Build history of the part. All positions in model axes, mm. A direction names the side the tool comes from. Give positions to 0.01 mm unless a question says otherwise; leave off trailing zeros. Order: outer loops, then holes, each group sorted by start corner. A loop starts at its lowest first (then second) coordinate and runs counter-clockwise, first axis right, second up. Notation, with made-up numbers: (30.5, 46) - (61.5, 46) arc R21 cw to (61.5, 77) - close; hole circle Ø6 at (-24.5, 29.5). An arc over 180 degrees is marked (long way). One line per item, written item: value.
```python
from build123d import *

# Parameters (mm, degrees)
CYLINDER063_R              = 1.6
CYLINDER063_DEPTH          = 10
EXTRUDE027_DEPTH           = 6
EXTRUDE030_DEPTH           = 6
EXTRUDE030_PLACEMENT_ANGLE = 180
CYLINDER072_R              = 1.5
CYLINDER072_DEPTH          = 45
PRISM011_DEPTH             = 3
CYLINDER071_R              = 3
CYLINDER071_DEPTH          = 5
FUSION063_PLACEMENT_ANGLE  = 180
CYLINDER070_R              = 1.5
CYLINDER070_DEPTH          = 45
PRISM010_DEPTH             = 3
CYLINDER068_R              = 3
CYLINDER068_DEPTH          = 5
EXTRUDE026_DEPTH           = 24
REVOLVE001_ANGLE           = 180
EXTRUDE025_DEPTH           = 74
FILLET004_R                = 2.5


with BuildPart() as cono003:
    # Cone003 → Cone003 (revolve)
    with BuildSketch(Plane(origin=(0, 0, -96), x_dir=(1, 0, 0), z_dir=(0, -1, 0))):
        Polygon((0, 0), (1.6, 0), (4.1, 3), (0, 3), align=None)
    revolve(axis=Axis((0, 0, -96), (0, 0, 1)))


with BuildPart() as cilindro063:
    # Cylinder063 → Cylinder063 (new body)
    with BuildSketch(Plane.XY.offset(-106)):
        Circle(CYLINDER063_R)
    extrude(amount=CYLINDER063_DEPTH)


with BuildPart() as fusion058:
    # Fusion058 base: copy of Cilindro063
    add(cilindro063.part)

    # Fusion058: union Cono003
    add(cono003.part)


with BuildPart() as fusion058_1:
    # Fusion058 placement: moved
    add(fusion058.part.moved(Location((65, 107, 0))))


with BuildPart() as fusion059:
    # Fusion057 base: copy of Cilindro063
    add(cilindro063.part)

    # Fusion057: union Cono003
    add(cono003.part)


with BuildPart() as fusion059_1:
    # Fusion057 placement: moved
    add(fusion059.part.moved(Location((-65, 107, 0))))

    # Fusion059: union Fusion058
    add(fusion058_1.part)


with BuildPart() as extrude027:
    # Sketch020 → Extrude027 (new body)
    with BuildSketch(Plane.XY.offset(-99)):
        with BuildLine():
            ThreePointArc((0, 10), (-10, 0), (0, -10))
            Line((20, -10), (0, -10))
            Line((20, 10), (20, -10))
            Line((0, 10), (20, 10))
        make_face()
    extrude(amount=EXTRUDE027_DEPTH)


with BuildPart() as extrude027_1:
    # Extrude027 placement: moved
    add(extrude027.part.moved(Location((-65, 107, 0))))


with BuildPart() as cut022:
    # Sketch020 → Extrude030 (new body)
    with BuildSketch(Plane.XY.offset(-99)):
        with BuildLine():
            ThreePointArc((0, 10), (-10, 0), (0, -10))
            Line((20, -10), (0, -10))
            Line((20, 10), (20, -10))
            Line((0, 10), (20, 10))
        make_face()
    extrude(amount=EXTRUDE030_DEPTH)


with BuildPart() as cut022_1:
    # Extrude030 placement: moved
    add(cut022.part.moved(Location((65, 107, 0))).rotate(Axis((65, 107, 0), (0, 0, 1)), EXTRUDE030_PLACEMENT_ANGLE))

    # Fusion055: union Extrude027
    add(extrude027_1.part)

    # Cut022: cut Fusion059
    add(fusion059_1.part, mode=Mode.SUBTRACT)


with BuildPart() as cilindro072:
    # Cylinder072 → Cylinder072 (new body)
    with BuildSketch(Plane(origin=(33, 0, -87), x_dir=(0, 0, 1), z_dir=(-1, 0, 0))):
        Circle(CYLINDER072_R)
    extrude(amount=CYLINDER072_DEPTH)


with BuildPart() as prisma011:
    # Prism011 → Prism011 (new body)
    with BuildSketch(Plane(origin=(0, 0, -87), x_dir=(0, 0, 1), z_dir=(-1, 0, 0))):
        Polygon((3, 0), (1.5, 2.598076), (-1.5, 2.598076), (-3, 0), (-1.5, -2.598076), (1.5, -2.598076), align=None)
    extrude(amount=PRISM011_DEPTH)


with BuildPart() as fusion063:
    # Cylinder071 → Cylinder071 (new body)
    with BuildSketch(Plane(origin=(24, 0, -87), x_dir=(0, 0, 1), z_dir=(-1, 0, 0))):
        Circle(CYLINDER071_R)
    extrude(amount=CYLINDER071_DEPTH)

    # Fusion063: union Cilindro072, Prisma011
    add(cilindro072.part)
    add(prisma011.part)


with BuildPart() as fusion063_1:
    # Fusion063 placement: moved
    add(fusion063.part.moved(Location((-65, 36, 0))).rotate(Axis((-65, 36, 0), (0, 0, 1)), FUSION063_PLACEMENT_ANGLE))


with BuildPart() as cilindro070:
    # Cylinder070 → Cylinder070 (new body)
    with BuildSketch(Plane(origin=(98, 36, -87), x_dir=(0, 0, 1), z_dir=(-1, 0, 0))):
        Circle(CYLINDER070_R)
    extrude(amount=CYLINDER070_DEPTH)


with BuildPart() as prisma010:
    # Prism010 → Prism010 (new body)
    with BuildSketch(Plane(origin=(65, 36, -87), x_dir=(0, 0, 1), z_dir=(-1, 0, 0))):
        Polygon((3, 0), (1.5, 2.598076), (-1.5, 2.598076), (-3, 0), (-1.5, -2.598076), (1.5, -2.598076), align=None)
    extrude(amount=PRISM010_DEPTH)


with BuildPart() as fusion061:
    # Cylinder068 → Cylinder068 (new body)
    with BuildSketch(Plane(origin=(89, 36, -87), x_dir=(0, 0, 1), z_dir=(-1, 0, 0))):
        Circle(CYLINDER068_R)
    extrude(amount=CYLINDER068_DEPTH)

    # Fusion062: union Cilindro070, Prisma010
    add(cilindro070.part)
    add(prisma010.part)

    # Fusion061: union Fusion063
    add(fusion063_1.part)


with BuildPart() as cut023:
    # Sketch019 → Extrude026 (new body)
    with BuildSketch(Plane.XY.offset(-75)):
        with BuildLine():
            ThreePointArc((-48, 117), (-67.384986, 70.729267), (-74, 21))
            Line((-74, 21), (-74, 0))
            Line((-74, 0), (74, 0))
            Line((74, 21), (74, 0))
            ThreePointArc((74, 21), (67.384986, 70.729267), (48, 117))
            Line((-48, 117), (48, 117))
        make_face()
        with BuildLine():
            Line((-38, 107), (-7.5, 107))
            Line((-7.5, 107), (-7.5, 7.5))
            Line((-7.5, 7.5), (-64, 7.5))
            Line((-64, 7.5), (-64, 21))
            ThreePointArc((-38, 107), (-57.357897, 65.922155), (-64, 21))
        make_face(mode=Mode.SUBTRACT)
        with BuildLine():
            Line((7.5, 107), (7.5, 7.5))
            Line((7.5, 7.5), (64, 7.5))
            Line((64, 7.5), (64, 21))
            ThreePointArc((64, 21), (57.357897, 65.922155), (38, 107))
            Line((38, 107), (7.5, 107))
        make_face(mode=Mode.SUBTRACT)
    extrude(amount=-EXTRUDE026_DEPTH)

    # Cut023: cut Fusion061
    add(fusion061.part, mode=Mode.SUBTRACT)


with BuildPart() as revolve001:
    # Sketch017 → Revolve001 (revolve)
    with BuildSketch(Plane.XY):
        with BuildLine():
            Line((-65, 21), (-65, -21))
            ThreePointArc((-65, -21), (-58.133531, -73.27332), (-38, -122))
            Line((-38, -122), (0, -122))
            Line((0, 122), (0, -122))
            Line((0, 122), (-38, 122))
            ThreePointArc((-38, 122), (-58.133531, 73.27332), (-65, 21))
        make_face()
    revolve(axis=Axis((0, 0, 0), (0, -1, 0)), revolution_arc=REVOLVE001_ANGLE)


with BuildPart() as obj1:
    # Sketch018 → Extrude025 (new body)
    with BuildSketch(Plane.XY):
        with BuildLine():
            Line((-74, 21), (-74, 0))
            Line((-74, 0), (74, 0))
            Line((74, 21), (74, 0))
            ThreePointArc((74, 21), (67.384986, 70.729267), (48, 117))
            Line((-48, 117), (48, 117))
            ThreePointArc((-48, 117), (-67.384986, 70.729267), (-74, 21))
        make_face()
    extrude(amount=-EXTRUDE025_DEPTH)


with BuildPart() as obj1_1:
    # Extrude025 placement: moved
    add(obj1.part.moved(Location((0, 0, -1))))

    # Cut021: cut Revolve001
    add(revolve001.part, mode=Mode.SUBTRACT)

    # Fillet004
    fillet004_edges = [obj1_1.edges().sort_by_distance(p)[0] for p in [
        (67.384986, 70.729267, -1),
        (74, 10.5, -1),
        (44.386684, 117, -1),
        (0, 117, -40.78563),
        (-44.386684, 117, -1),
        (64.992307, 10.5, -1),
        (58.844411, 70.504014, -1),
        (-58.844411, 70.504014, -1),
        (-64.992307, 10.5, -1),
        (-74, 10.5, -1),
        (-67.384986, 70.729267, -1),
    ]]
    fillet(fillet004_edges, radius=FILLET004_R)

    # Fusion060: union Cut022, Cut023
    add(cut022_1.part)
    add(cut023.part)


solid = obj1_1.part
```
(1) Pin check, flat tips, straight feed: P1, Ø2, axis at x = -56.5, z = -86.5, coming from the +Y side; P2, Ø4, axis at x = 27, y = 30, coming from the -Z side; P3, Ø15, axis at y = 12, z = -86.5, coming from the -X side. Stop position of each tip, or through.
Completed:
P1: y = 102.83
P2: z = -75
P3: x = -74
(2) 3-axis set-ups, long thin cutter, end or side, ignore diameter. For faces 4 (the face through (75, 107, -96)), 5 (the face through (-23, 107, -87)), 6 (the face through (62, 111, -93)), 7 (the face through (-62, 97, -96)): which of +Z, -Z, +X, -X, +Y, -Y reach the whole face in a straight line?
Completed:
face 4: +Z, -Z, +X
face 5: -Z
face 6: +Z, +X, +Y
face 7: +Z, -Z, -X
(3) Pull direction X, two halves, no side cores. Call faces 1 (the face through (-1.382, 10.353, -64.985)), 2 (the face through (62, 97, -96)), 3 (the face through (-75, 107, -96)): +X half, -X half, draft (parallel to the pull), parting line (faces both ways), or undercut.
Completed:
face 1: undercut
face 2: draft
face 3: -X half
(4) Slice it at A-A, the plane z = -73. Give the cut face in (x, y), and give its area (3 significant figures).
Completed:
outline: (-74, 0) - (74, 0) - (74, 21) arc R190.23 ccw to (48, 117) - (-48, 117) arc R190.23 ccw to (-74, 21) - close
area: 15,700 mm²
(5) Drill centre lines: line 1 (X direction, y = 10, z = -81); line 2 (Z direction, x = 70.25, y = 36); line 3 (X direction, y = 42.5, z = -83.5). Where is each one in solid material? Low to high.
Completed:
line 1: -74 to -64, -7.5 to 7.5, 64 to 74
line 2: -99 to -88.5, -85.5 to -1
line 3: -72.78 to -62.5, -7.5 to 7.5, 62.5 to 72.78
